The model under review builds one solid part; all positions refer to its coordinate system, in mm. A direction names the side the tool comes from. Round coordinates to 2 decimals unless told otherwise and drop trailing zeros. Order: outer loops, then holes, each group sorted by start corner. A loop starts at its lowest first (then second) coordinate and runs counter-clockwise, first axis right, second up. Notation, with made-up numbers: (43.5, 37.5) -> (72.5, 37.5) arc R23 cw to (72.5, 52.5) -> close; hole circle Ø6 at (-39.5, -27.75). An arc over 180 degrees is marked (long way). Use a Markdown table: item, result. Add a question column.
```python
from build123d import *

# Parameters (mm, degrees)
F1_DEPTH = 25
F3_DEPTH = 1


with BuildPart() as f1:
    # F0 (on Top) → F1 (new body)
    with BuildSketch(Plane.XY):
        with BuildLine():
            Line((22.6195406914, 28.6195406914), (-22.6195406914, 28.6195406914))
            ThreePointArc((-22.6195406914, 28.6195406914), (-26.8621813785, 26.8621813785), (-28.6195406914, 22.6195406914))
            Line((-28.6195406914, 22.6195406914), (-28.6195406914, -22.6195406914))
            ThreePointArc((-28.6195406914, -22.6195406914), (-26.8621813785, -26.8621813785), (-22.6195406914, -28.6195406914))
            Line((-22.6195406914, -28.6195406914), (22.6195406914, -28.6195406914))
            ThreePointArc((22.6195406914, -28.6195406914), (26.8621813785, -26.8621813785), (28.6195406914, -22.6195406914))
            Line((28.6195406914, -22.6195406914), (28.6195406914, 22.6195406914))
            ThreePointArc((28.6195406914, 22.6195406914), (26.8621813785, 26.8621813785), (22.6195406914, 28.6195406914))
        make_face()
        with BuildLine():
            ThreePointArc((-27.6195406914, 22.6195406914), (-26.1550745973, 26.1550745973), (-22.6195406914, 27.6195406914))
            Line((-22.6195406914, 27.6195406914), (22.6195406914, 27.6195406914))
            ThreePointArc((22.6195406914, 27.6195406914), (26.1550745973, 26.1550745973), (27.6195406914, 22.6195406914))
            Line((27.6195406914, 22.6195406914), (27.6195406914, -22.6195406914))
            ThreePointArc((27.6195406914, -22.6195406914), (26.1550745973, -26.1550745973), (22.6195406914, -27.6195406914))
            Line((22.6195406914, -27.6195406914), (-22.6195406914, -27.6195406914))
            ThreePointArc((-22.6195406914, -27.6195406914), (-26.1550745973, -26.1550745973), (-27.6195406914, -22.6195406914))
            Line((-27.6195406914, -22.6195406914), (-27.6195406914, 22.6195406914))
        make_face(mode=Mode.SUBTRACT)
    extrude(amount=F1_DEPTH)

    # F2 (on face) → F3 (join)
    with BuildSketch(Plane.XY.offset(25)):
        with BuildLine():
            ThreePointArc((22.6195406914, -28.6195406914), (26.8621813785, -26.8621813785), (28.6195406914, -22.6195406914))
            Line((28.6195406914, -22.6195406914), (28.6195406914, 22.6195406914))
            ThreePointArc((28.6195406914, 22.6195406914), (26.8621813785, 26.8621813785), (22.6195406914, 28.6195406914))
            Line((22.6195406914, 28.6195406914), (-22.6195406914, 28.6195406914))
            ThreePointArc((-22.6195406914, 28.6195406914), (-26.8621813785, 26.8621813785), (-28.6195406914, 22.6195406914))
            Line((-28.6195406914, 22.6195406914), (-28.6195406914, -22.6195406914))
            ThreePointArc((-28.6195406914, -22.6195406914), (-26.8621813785, -26.8621813785), (-22.6195406914, -28.6195406914))
            Line((-22.6195406914, -28.6195406914), (22.6195406914, -28.6195406914))
        make_face()
        with BuildLine():
            Line((-27.6195406914, -22.6195406914), (-27.6195406914, 22.6195406914))
            ThreePointArc((-27.6195406914, 22.6195406914), (-26.1550745973, 26.1550745973), (-22.6195406914, 27.6195406914))
            Line((-22.6195406914, 27.6195406914), (22.6195406914, 27.6195406914))
            ThreePointArc((22.6195406914, 27.6195406914), (26.1550745973, 26.1550745973), (27.6195406914, 22.6195406914))
            Line((27.6195406914, 22.6195406914), (27.6195406914, -22.6195406914))
            ThreePointArc((27.6195406914, -22.6195406914), (26.1550745973, -26.1550745973), (22.6195406914, -27.6195406914))
            Line((22.6195406914, -27.6195406914), (-22.6195406914, -27.6195406914))
            ThreePointArc((-22.6195406914, -27.6195406914), (-26.1550745973, -26.1550745973), (-27.6195406914, -22.6195406914))
        make_face(mode=Mode.SUBTRACT)
        with BuildLine():
            ThreePointArc((-22.6195406914, 27.6195406914), (-26.1550745973, 26.1550745973), (-27.6195406914, 22.6195406914))
            Line((-27.6195406914, 22.6195406914), (-27.6195406914, -22.6195406914))
            ThreePointArc((-27.6195406914, -22.6195406914), (-26.1550745973, -26.1550745973), (-22.6195406914, -27.6195406914))
            Line((-22.6195406914, -27.6195406914), (22.6195406914, -27.6195406914))
            ThreePointArc((22.6195406914, -27.6195406914), (26.1550745973, -26.1550745973), (27.6195406914, -22.6195406914))
            Line((27.6195406914, -22.6195406914), (27.6195406914, 22.6195406914))
            ThreePointArc((27.6195406914, 22.6195406914), (26.1550745973, 26.1550745973), (22.6195406914, 27.6195406914))
            Line((22.6195406914, 27.6195406914), (-22.6195406914, 27.6195406914))
        make_face()
    extrude(amount=F3_DEPTH)


solid = f1.part
```
Q1. Insertion check: pin 1 (10 mm diameter, centred on x = 11.5, y = -4.5, fed in from -Z). The pin has a flat end and moves straight along its axis. Give the tip position at first contact, or say it passes through.
Q2. Add section A-A (y = 11.5). Write out the cut boundary in (x, z), then the cut area to 3 significant figures.
Q3. Mouldability with a two-part tool opening along Y and no side actions: class faces 3 (the flat face through (0, 0, 26)), 4 (the flat face through (27.62, 0, 12)), 5 (the cylindrical face through (26.815, -26.909, 12.818)) as pulls with the +Y half, pulls with the -Y half, needs draft (parallel to the pull), parting line crosses it, or undercut.
Q4. Wall thickness on line 1 (Y direction, x = 8, z = 11.5); line 2 (Z direction, x = -23, y = -22.5): over which ranges is each line inside the solid? List them lowest first. Write a range as [from, to].
Q5. Machinability: for faces 1 (the cylindrical face through (-26.909, -26.815, 12.818)), 2 (the flat face through (-27.62, 0, 12)), which of the approach directions +Z, -Z, +X, -X, +Y, -Y give a long, thin tool a straight path to every point of the face, cutting with its end or side? Answer none if there is none.
Q6. Add section B-B (z = 20.75). Write out the cut boundary in (x, y), then the cut area to 3 significant figures.
Report:
| question | item | result |
|---|---|---|
| 1 | pin 1 | stops at z = 25 |
| 2 | outline | (-28.62, 0) -> (-27.62, 0) -> (-27.62, 25) -> (27.62, 25) -> (27.62, 0) -> (28.62, 0) -> (28.62, 26) -> (-28.62, 26) -> close |
| 2 | area | 107 mm² |
| 3 | face 3 | needs draft |
| 3 | face 4 | undercut |
| 3 | face 5 | pulls with the -Y half |
| 4 | line 1 | y = [-28.62, -27.62], [27.62, 28.62] |
| 4 | line 2 | z = [25, 26] |
| 5 | face 1 | +Z, -Z, -X, -Y |
| 5 | face 2 | -Z |
| 6 | outline | (-28.62, -22.62) arc R6 ccw to (-22.62, -28.62) -> (22.62, -28.62) arc R6 ccw to (28.62, -22.62) -> (28.62, 22.62) arc R6 ccw to (22.62, 28.62) -> (-22.62, 28.62) arc R6 ccw to (-28.62, 22.62) -> close; hole (-27.62, -22.62) arc R5 ccw to (-22.62, -27.62) -> (22.62, -27.62) arc R5 ccw to (27.62, -22.62) -> (27.62, 22.62) arc R5 ccw to (22.62, 27.62) -> (-22.62, 27.62) arc R5 ccw to (-27.62, 22.62) -> close |
| 6 | area | 216 mm² |
